```python
from build123d import *

# Parameters (mm, degrees)
ESQUISSE1_W        = 23
ESQUISSE1_H        = 12
BOSS_EXTRU_1_DEPTH = 22
ESQUISSE2_R        = 2.5
ESQUISSE2_R_2      = 6
BOSS_EXTRU_2_DEPTH = 5
ESQUISSE3_R        = 2.5
BOSS_EXTRU_3_DEPTH = 3
ESQUISSE4_W        = 2.5
ESQUISSE4_H        = 12
BOSS_EXTRU_4_DEPTH = 5


with BuildPart() as part:
    # Esquisse1 → Boss.-Extru.1 (new body)
    with BuildSketch(Plane.XY):
        Rectangle(ESQUISSE1_W, ESQUISSE1_H)
    extrude(amount=BOSS_EXTRU_1_DEPTH)

    # Esquisse2 → Boss.-Extru.2 (add)
    with BuildSketch(Plane.XY.offset(22)):
        Circle(ESQUISSE2_R)
        with Locations((-5.5, 0)):
            Circle(ESQUISSE2_R_2)
    extrude(amount=BOSS_EXTRU_2_DEPTH)

    # Esquisse3 → Boss.-Extru.3 (add)
    with BuildSketch(Plane.XY.offset(27)):
        with Locations((-5.5, 0)):
            Circle(ESQUISSE3_R)
    extrude(amount=BOSS_EXTRU_3_DEPTH)

    # Esquisse4 → Boss.-Extru.4 (add)
    with BuildSketch(Plane.ZY.offset(11.5)):
        with Locations((17.25, 0)):
            Rectangle(ESQUISSE4_W, ESQUISSE4_H)
    boss_extru_4 = extrude(amount=BOSS_EXTRU_4_DEPTH)

    # Symétrie1: Boss.-Extru.4 across plane
    add(boss_extru_4.mirror(Plane(origin=(0, 0, 0), x_dir=(0, 0, 1), z_dir=(1, 0, 0))))


solid = part.part
```
For this review, take the finished solid that the model builds, in its own axes (mm). A direction names the side the tool comes from. Round coordinates to 2 decimals unless told otherwise and drop trailing zeros. Order: outer loops, then holes, each group sorted by start corner. A loop starts at its lowest first (then second) coordinate and runs counter-clockwise, first axis right, second up. Notation, with made-up numbers: (29.25, 56) -> (69.25, 56) arc R6 cw to (69.25, 60) -> close; hole circle Ø5 at (-14, 69.25). An arc over 180 degrees is marked (long way). Use a Markdown table: item, result.
Item 1: Take a section at D-D (x = -7.5). State the section outline as (y, z) points.
Resolved:
| item | result |
|---|---|
| outline | (-6, 0) -> (6, 0) -> (6, 22) -> (5.66, 22) -> (5.66, 27) -> (1.5, 27) -> (1.5, 30) -> (-1.5, 30) -> (-1.5, 27) -> (-5.66, 27) -> (-5.66, 22) -> (-6, 22) -> close |
Item 2: Take a section at C-C (z = 15). State the section outline as (x, y) points, plus the area to 3 significant figures.
Resolved:
| item | result |
|---|---|
| outline | (-11.5, -6) -> (11.5, -6) -> (11.5, 6) -> (-11.5, 6) -> close |
| area | 276 mm² |
Item 3: Take a section at A-A (y = -3.75). State the section outline as (x, z) points.
Resolved:
| item | result |
|---|---|
| outline | (-16.5, 16) -> (-11.5, 16) -> (-11.5, 0) -> (11.5, 0) -> (11.5, 16) -> (16.5, 16) -> (16.5, 18.5) -> (11.5, 18.5) -> (11.5, 22) -> (-0.82, 22) -> (-0.82, 27) -> (-10.18, 27) -> (-10.18, 22) -> (-11.5, 22) -> (-11.5, 18.5) -> (-16.5, 18.5) -> close |
Item 4: Take a section at B-B (x = 11). State the section outline as (y, z) points.
Resolved:
| item | result |
|---|---|
| outline | (-6, 0) -> (6, 0) -> (6, 22) -> (-6, 22) -> close |
Item 5: Machinability: for faces 1 (the flat face through (14, 0, 16)), 2 (the flat face through (-10, -5, 22)), 3 (the flat face through (-14, 0, 16)), which of the approach directions +Z, -Z, +X, -X, +Y, -Y give a long, thin tool a straight path to every point of the face, cutting with its end or side? Answer none if there is none.
Resolved:
| item | result |
|---|---|
| face 1 | -Z, +X, +Y, -Y |
| face 2 | +Z, -X, -Y |
| face 3 | -Z, -X, +Y, -Y |
Item 6: For pin 1 (3 mm diameter, centred on x = 7.5, y = -1, fed in from +Z); pin 2 (2.5 mm diameter, centred on x = 14.5, y = -1, fed in from +Z); pin 3 (2 mm diameter, centred on x = -6, y = -4, fed in from +Z), all flat-tipped, find the tip position at first contact; note any pin that passes through.
Resolved:
| item | result |
|---|---|
| pin 1 | stops at z = 22 |
| pin 2 | stops at z = 18.5 |
| pin 3 | stops at z = 27 |
Item 7: For line 1 along Z through (x, y) = (-13, -1.5); line 2 along Z through (x, y) = (5.5, -1.5); line 3 along X through (y, z) = (-2, 12.5), list the stretches that pass through material, from the lowest coordinate up. Write a range as [from, to].
Resolved:
| item | result |
|---|---|
| line 1 | z = [16, 18.5] |
| line 2 | z = [0, 22] |
| line 3 | x = [-11.5, 11.5] |
